Study the drawing (mm; zero at the part's minimum x, y, z) and answer. A direction names the side the tool comes from. Give positions to 0.01 mm unless a question says otherwise; leave off trailing zeros. Write each loop counter-clockwise with the first axis right and the second up, starting at its lowest first coordinate (ties: lowest second). Pieces come first, ordered by that corner, then holes. Notation, with made-up numbers: (75.5, -20.75) - (128.5, -20.75) arc R29 ccw to (128.5, 14.25) - close; hole circle Ø4 at (19, 89). An arc over 180 degrees is marked (long way). Answer as CSV lines item,"result".
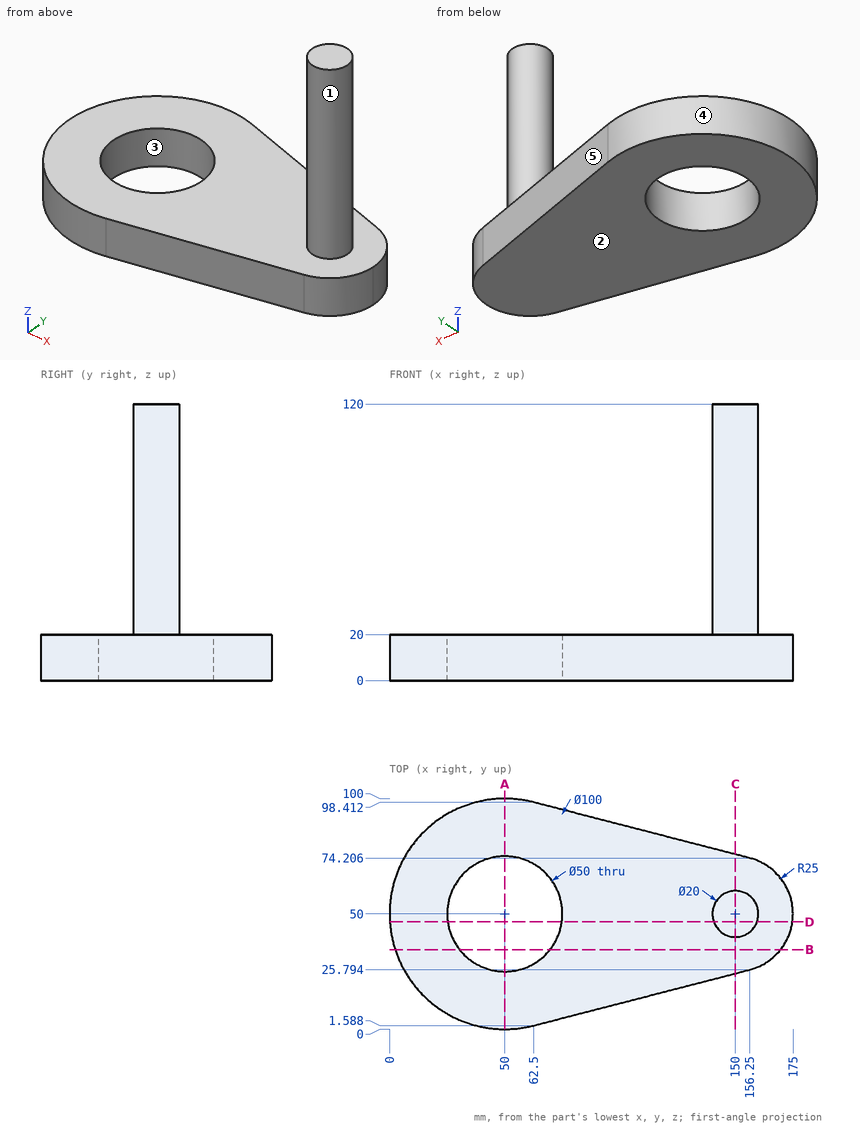
(1) The mould has two halves that part along Y. Classify the marked faces 3, 4 and 5: +Y half, -Y half, draft (parallel to the pull), parting line (faces both ways), or undercut.
Worked out:
face 3,"undercut"
face 4,"parting line"
face 5,"+Y half"
(2) This flat-tipped pin is pushed along its axis until it touches: P1, Ø10, axis at x = 127, y = 29.5, coming from the +Z side. Where does it stop, or does it pass through?
Worked out:
P1,"stops at z = 20"
(3) A cutting plane is placed at B-B (y = 34.5). Write down the section's boundary in (x, z) (1 decimal), and give its area (3 significant figures).
Worked out:
outline,"(2.5, 0) - (30.4, 0) - (30.4, 20) - (2.5, 20) - close; (69.6, 0) - (169.6, 0) - (169.6, 20) - (69.6, 20) - close"
area,"2,560 mm^2"
(4) A cutting plane is placed at D-D (y = 46.5). Write down the section's boundary in (x, z).
Worked out:
outline,"(0.12, 0) - (25.25, 0) - (25.25, 20) - (0.12, 20) - close; (74.75, 0) - (174.75, 0) - (174.75, 20) - (159.37, 20) - (159.37, 120) - (140.63, 120) - (140.63, 20) - (74.75, 20) - close"
(5) A cutting plane is placed at C-C (x = 150). Write down the section's boundary in (y, z).
Worked out:
outline,"(24.18, 0) - (75.82, 0) - (75.82, 20) - (60, 20) - (60, 120) - (40, 120) - (40, 20) - (24.18, 20) - close"
(6) For the marked faces 1 and 2, determine the directions among +Z, -Z, +X, -X, +Y, -Y from which every point of the face is accessible in a straight line to the end or side of a thin tool.
Worked out:
face 1,"+Z"
face 2,"-Z, +X, -X, +Y, -Y"
(7) Find the intervals of material crossed by L1, parallel to Y at x = 50, z = 7; L2, parallel to Z at x = 86, y = 72; L3, parallel to X at y = 29, z = 16.5 (1 decimal), in increasing order.
Worked out:
L1,"y = 0 to 25, 75 to 100"
L2,"z = 0 to 20"
L3,"x = 4.6 to 36.4, 63.6 to 163.6"
(8) A cutting plane is placed at A-A (x = 50). Write down the section's boundary in (y, z), and give its area (3 significant figures).
Worked out:
outline,"(0, 0) - (25, 0) - (25, 20) - (0, 20) - close; (75, 0) - (100, 0) - (100, 20) - (75, 20) - close"
area,"1,000 mm^2"
